Work out the finished part from the listing and answer in its coordinate system (mm). A direction names the side the tool comes from. Round coordinates to 2 decimals unless told otherwise and drop trailing zeros. Write each loop counter-clockwise with the first axis right and the second up, starting at its lowest first coordinate (ties: lowest second). Pieces come first, ordered by that corner, then holes. Notation, with made-up numbers: M -24,-3.5 L 12,-3.5 A33 ccw 12,29.5 Z; hole C -25,89 d5. An arc over 180 degrees is marked long. One line per item, written item: value. Start each with the question number.
Q1. A tool of negligible diameter and unlimited length cuts with its end or side. For faces 1 (the cylindrical face through (49.19, 15.95, 19.53)), 2 (the flat face through (-1, 41.275, 33)), 3 (the cylindrical face through (-47.18, 40.63, 32.19)), from which of +Z, -Z, +X, -X, +Y, -Y can it reach the whole face along a straight path? Write none if from no direction.
Q2. Find section B-B (x = -18). Write down the section's boundary in (y, z) (3 decimals).
Q3. Find section C-C (y = 17.5). Write down the section's boundary in (x, z) (3 decimals).
Q4. Find section D-D (y = -20.5). Write down the section's boundary in (x, z) (3 decimals).
Q5. The mould has two halves that part along X. Classify faces 4 (the flat face through (-1, 1, 3.175)), 5 (the flat face through (0, 43, 63.5)), 6 (the flat face through (53.975, 20, 18)), 7 (the cylindrical face through (-44.91, -38.41, 33.76)): released by +X, released by -X, zero draft, split by the parting line, or undercut.
Q6. Find section A-A (z = 26.5). Write down the section's boundary in (x, y) (3 decimals).
Q7. Given pin 1 Ø3.5 at (y, z) = (16.5, 19) entering from +X (3 decimals); pin 2 Ø10 at (x, y) = (36.5, 14) entering from +Z (3 decimals), each flat-ended and moving along its own axis, determine where each tip first touches the part or whether it passes through.
Q8. Consider probe 1 along Y at (x, z) = (9, 8) (3 decimals); probe 2 along X at (y, z) = (15.5, 33.5) (3 decimals); probe 3 along Z at (x, y) = (-32.5, -36) (3 decimals). Determine where each line is inside the solid, lowest interval first.
from build123d import *

# Parameters (mm, degrees)
F5_W     = 101.6
F5_H     = 88.9
F6_DEPTH = 63.5
F0_R     = 12.7
F1_T     = -3.175
F2_D     = 3.175
F2_DEPTH = 12.7
F3_R     = 3.175
F3_R_2   = 2.12725
F4_DEPTH = 3.175


with BuildPart() as f6:
    # F5 (on Top) → F6 (new body)
    with BuildSketch(Plane.XY):
        Rectangle(F5_W, F5_H)
    extrude(amount=F6_DEPTH)

    # F0
    f0_edges = [f6.edges().sort_by_distance(p)[0] for p in [
        (50.8, -44.45, 31.75),
        (50.8, 44.45, 31.75),
        (-50.8, -44.45, 31.75),
        (-50.8, 44.45, 31.75),
    ]]
    fillet(f0_edges, radius=F0_R)

    # F1
    f1_openings = [f6.faces().sort_by_distance(p)[0] for p in [
        (0, 0, 63.5),
    ]]
    offset(amount=F1_T, openings=f1_openings)

    # F2
    with Locations(Plane.YZ.offset(50.8)):
        with Locations((17.4625, 19.05)):
            Hole(F2_D / 2, depth=F2_DEPTH)

    # F3 (on face) → F4 (join)
    with BuildSketch(Plane.YZ.offset(50.8)):
        with Locations((17.4625, 19.05)):
            Circle(F3_R)
        with Locations((17.4625, 19.05)):
            Circle(F3_R_2, mode=Mode.SUBTRACT)
    extrude(amount=F4_DEPTH)


solid = f6.part
The answers:
1. face 1: +X
1. face 2: +Z
1. face 3: +Z, -Z, -X, +Y
2. outline: M -44.45,0 L 44.45,0 L 44.45,63.5 L 41.275,63.5 L 41.275,3.175 L -41.275,3.175 L -41.275,63.5 L -44.45,63.5 Z
3. outline: M -50.8,0 L 50.8,0 L 50.8,15.875 L 53.975,15.875 L 53.975,16.923 L 50.8,16.923 L 50.8,17.463 L 47.625,17.463 L 47.625,3.175 L -47.625,3.175 L -47.625,63.5 L -50.8,63.5 Z; M 47.625,20.637 L 50.8,20.637 L 50.8,21.177 L 53.975,21.177 L 53.975,22.225 L 50.8,22.225 L 50.8,63.5 L 47.625,63.5 Z
4. outline: M -50.8,0 L 50.8,0 L 50.8,63.5 L 47.625,63.5 L 47.625,3.175 L -47.625,3.175 L -47.625,63.5 L -50.8,63.5 Z
5. face 4: undercut
5. face 5: zero draft
5. face 6: released by +X
5. face 7: undercut
6. outline: M -50.8,-31.75 A12.7 ccw -38.1,-44.45 L 38.1,-44.45 A12.7 ccw 50.8,-31.75 L 50.8,31.75 A12.7 ccw 38.1,44.45 L -38.1,44.45 A12.7 ccw -50.8,31.75 Z; hole M -47.625,-31.75 A9.525 ccw -38.1,-41.275 L 38.1,-41.275 A9.525 ccw 47.625,-31.75 L 47.625,31.75 A9.525 ccw 38.1,41.275 L -38.1,41.275 A9.525 ccw -47.625,31.75 Z
7. pin 1: x = 53.975
7. pin 2: z = 3.175
8. probe 1: -44.45 to -41.275, 41.275 to 44.45
8. probe 2: -50.8 to -47.625, 47.625 to 50.8
8. probe 3: 0 to 3.175
